```python
from build123d import *

# Parameters (mm, degrees)
BOSS_EXTRUDE1_DEPTH = 261.8
CUT_EXTRUDE1_DEPTH  = 4001.062499512


with BuildPart() as part:
    # Sketch1 → Boss-Extrude1 (new body)
    with BuildSketch(Plane.XY.offset(4000)):
        with BuildLine():
            Line((10, 3.138), (10, 8.5))
            ThreePointArc((10, 8.5), (9.560660172, 9.560660172), (8.5, 10))
            Line((8.5, 10), (3.138, 10))
            ThreePointArc((3.138, 10), (2.778789755, 9.851210245), (2.63, 9.492))
            Line((2.63, 9.492), (2.63, 9.008))
            ThreePointArc((2.63, 9.008), (2.778789755, 8.648789755), (3.138, 8.5))
            Line((3.138, 8.5), (5.487, 8.5))
            ThreePointArc((5.487, 8.5), (5.846210245, 8.351210245), (5.995, 7.992))
            Line((5.995, 7.992), (5.995, 7.266080661))
            ThreePointArc((5.995, 7.266080661), (5.956330803, 7.071677478), (5.846210245, 6.906870417))
            Line((5.846210245, 6.906870417), (2.743129583, 3.803789755))
            ThreePointArc((2.743129583, 3.803789755), (2.578322522, 3.693669197), (2.383919339, 3.655))
            Line((2.383919339, 3.655), (-2.383919339, 3.655))
            ThreePointArc((-2.383919339, 3.655), (-2.578322522, 3.693669197), (-2.743129583, 3.803789755))
            Line((-2.743129583, 3.803789755), (-5.846210245, 6.906870417))
            ThreePointArc((-5.846210245, 6.906870417), (-5.956330803, 7.071677478), (-5.995, 7.266080661))
            Line((-5.995, 7.266080661), (-5.995, 7.992))
            ThreePointArc((-5.995, 7.992), (-5.846210245, 8.351210245), (-5.487, 8.5))
            Line((-5.487, 8.5), (-3.138, 8.5))
            ThreePointArc((-3.138, 8.5), (-2.778789755, 8.648789755), (-2.63, 9.008))
            Line((-2.63, 9.008), (-2.63, 9.492))
            ThreePointArc((-2.63, 9.492), (-2.778789755, 9.851210245), (-3.138, 10))
            Line((-3.138, 10), (-8.5, 10))
            ThreePointArc((-8.5, 10), (-9.560660172, 9.560660172), (-10, 8.5))
            Line((-10, 8.5), (-10, 3.138))
            ThreePointArc((-10, 3.138), (-9.851210245, 2.778789755), (-9.492, 2.63))
            Line((-9.492, 2.63), (-9.008, 2.63))
            ThreePointArc((-9.008, 2.63), (-8.648789755, 2.778789755), (-8.5, 3.138))
            Line((-8.5, 3.138), (-8.5, 5.487))
            ThreePointArc((-8.5, 5.487), (-8.351210245, 5.846210245), (-7.992, 5.995))
            Line((-7.992, 5.995), (-7.266080661, 5.995))
            ThreePointArc((-7.266080661, 5.995), (-7.071677478, 5.956330803), (-6.906870417, 5.846210245))
            Line((-6.906870417, 5.846210245), (-3.803789755, 2.743129583))
            ThreePointArc((-3.803789755, 2.743129583), (-3.693669197, 2.578322522), (-3.655, 2.383919339))
            Line((-3.655, 2.383919339), (-3.655, -2.383919339))
            ThreePointArc((-3.655, -2.383919339), (-3.693669197, -2.578322522), (-3.803789755, -2.743129583))
            Line((-3.803789755, -2.743129583), (-6.906870417, -5.846210245))
            ThreePointArc((-6.906870417, -5.846210245), (-7.071677478, -5.956330803), (-7.266080661, -5.995))
            Line((-7.266080661, -5.995), (-7.992, -5.995))
            ThreePointArc((-7.992, -5.995), (-8.351210245, -5.846210245), (-8.5, -5.487))
            Line((-8.5, -5.487), (-8.5, -3.138))
            ThreePointArc((-8.5, -3.138), (-8.648789755, -2.778789755), (-9.008, -2.63))
            Line((-9.008, -2.63), (-9.492, -2.63))
            ThreePointArc((-9.492, -2.63), (-9.851210245, -2.778789755), (-10, -3.138))
            Line((-10, -3.138), (-10, -8.5))
            ThreePointArc((-10, -8.5), (-9.560660172, -9.560660172), (-8.5, -10))
            Line((-8.5, -10), (-3.138, -10))
            ThreePointArc((-3.138, -10), (-2.778789755, -9.851210245), (-2.63, -9.492))
            Line((-2.63, -9.492), (-2.63, -9.008))
            ThreePointArc((-2.63, -9.008), (-2.778789755, -8.648789755), (-3.138, -8.5))
            Line((-3.138, -8.5), (-5.487, -8.5))
            ThreePointArc((-5.487, -8.5), (-5.846210245, -8.351210245), (-5.995, -7.992))
            Line((-5.995, -7.992), (-5.995, -7.266080661))
            ThreePointArc((-5.995, -7.266080661), (-5.956330803, -7.071677478), (-5.846210245, -6.906870417))
            Line((-5.846210245, -6.906870417), (-2.743129583, -3.803789755))
            ThreePointArc((-2.743129583, -3.803789755), (-2.578322522, -3.693669197), (-2.383919339, -3.655))
            Line((-2.383919339, -3.655), (2.383919339, -3.655))
            ThreePointArc((2.383919339, -3.655), (2.578322522, -3.693669197), (2.743129583, -3.803789755))
            Line((2.743129583, -3.803789755), (5.846210245, -6.906870417))
            ThreePointArc((5.846210245, -6.906870417), (5.956330803, -7.071677478), (5.995, -7.266080661))
            Line((5.995, -7.266080661), (5.995, -7.992))
            ThreePointArc((5.995, -7.992), (5.846210245, -8.351210245), (5.487, -8.5))
            Line((5.487, -8.5), (3.138, -8.5))
            ThreePointArc((3.138, -8.5), (2.778789755, -8.648789755), (2.63, -9.008))
            Line((2.63, -9.008), (2.63, -9.492))
            ThreePointArc((2.63, -9.492), (2.778789755, -9.851210245), (3.138, -10))
            Line((3.138, -10), (8.5, -10))
            ThreePointArc((8.5, -10), (9.560660172, -9.560660172), (10, -8.5))
            Line((10, -8.5), (10, -3.138))
            ThreePointArc((10, -3.138), (9.851210245, -2.778789755), (9.492, -2.63))
            Line((9.492, -2.63), (9.008, -2.63))
            ThreePointArc((9.008, -2.63), (8.648789755, -2.778789755), (8.5, -3.138))
            Line((8.5, -3.138), (8.5, -5.487))
            ThreePointArc((8.5, -5.487), (8.351210245, -5.846210245), (7.992, -5.995))
            Line((7.992, -5.995), (7.266080661, -5.995))
            ThreePointArc((7.266080661, -5.995), (7.071677478, -5.956330803), (6.906870417, -5.846210245))
            Line((6.906870417, -5.846210245), (3.803789755, -2.743129583))
            ThreePointArc((3.803789755, -2.743129583), (3.693669197, -2.578322522), (3.655, -2.383919339))
            Line((3.655, -2.383919339), (3.655, 2.383919339))
            ThreePointArc((3.655, 2.383919339), (3.693669197, 2.578322522), (3.803789755, 2.743129583))
            Line((3.803789755, 2.743129583), (6.906870417, 5.846210245))
            ThreePointArc((6.906870417, 5.846210245), (7.071677478, 5.956330803), (7.266080661, 5.995))
            Line((7.266080661, 5.995), (7.992, 5.995))
            ThreePointArc((7.992, 5.995), (8.351210245, 5.846210245), (8.5, 5.487))
            Line((8.5, 5.487), (8.5, 3.138))
            ThreePointArc((8.5, 3.138), (8.648789755, 2.778789755), (9.008, 2.63))
            Line((9.008, 2.63), (9.492, 2.63))
            ThreePointArc((9.492, 2.63), (9.851210245, 2.778789755), (10, 3.138))
        make_face()
        with BuildLine():
            Line((-2.124900844, -2.304505966), (-2.304505966, -2.124900844))
            ThreePointArc((-2.304505966, -2.124900844), (-2.505938017, -1.356467811), (-1.935133506, -0.803976718))
            ThreePointArc((-1.935133506, -0.803976718), (-2.0955, 0), (-1.935133506, 0.803976718))
            ThreePointArc((-1.935133506, 0.803976718), (-2.505938017, 1.356467811), (-2.304505966, 2.124900844))
            Line((-2.304505966, 2.124900844), (-2.124900844, 2.304505966))
            ThreePointArc((-2.124900844, 2.304505966), (-1.356467811, 2.505938017), (-0.803976718, 1.935133506))
            ThreePointArc((-0.803976718, 1.935133506), (0, 2.0955), (0.803976718, 1.935133506))
            ThreePointArc((0.803976718, 1.935133506), (1.356467811, 2.505938017), (2.124900844, 2.304505966))
            Line((2.124900844, 2.304505966), (2.304505966, 2.124900844))
            ThreePointArc((2.304505966, 2.124900844), (2.505938017, 1.356467811), (1.935133506, 0.803976718))
            ThreePointArc((1.935133506, 0.803976718), (2.0955, 0), (1.935133506, -0.803976718))
            ThreePointArc((1.935133506, -0.803976718), (2.505938017, -1.356467811), (2.304505966, -2.124900844))
            Line((2.304505966, -2.124900844), (2.124900844, -2.304505966))
            ThreePointArc((2.124900844, -2.304505966), (1.356467811, -2.505938017), (0.803976718, -1.935133506))
            ThreePointArc((0.803976718, -1.935133506), (0, -2.0955), (-0.803976718, -1.935133506))
            ThreePointArc((-0.803976718, -1.935133506), (-1.356467811, -2.505938017), (-2.124900844, -2.304505966))
        make_face(mode=Mode.SUBTRACT)
    extrude(amount=-BOSS_EXTRUDE1_DEPTH)

    # Sketch2 → Cut-Extrude1 (cut, through all)
    with BuildSketch(Plane.XZ.offset(10)):
        Polygon((10, 4000), (-10, 3995.213189756), (-10, 4000), align=None)
        Polygon((10, 3738.2), (10, 3742.986810244), (-10, 3738.2), align=None)
    extrude(amount=-CUT_EXTRUDE1_DEPTH, mode=Mode.SUBTRACT)


solid = part.part
```
Source: CAD feature listing. Evaluate the final solid. Frame: model axes, mm. A direction names the side the tool comes from. Round coordinates to 2 decimals unless told otherwise and drop trailing zeros. Use a Markdown table: item, result. Add a question column.
1. Ray query, line 1 along X through (y, z) = (-4.75, 3887); line 2 along Y through (x, z) = (1, 3956) (3 decimals); line 3 along X through (y, z) = (-8, 3987). Return the intervals inside material, ascending. Write a range as [from, to].
2. Contact query for flat-ended pins moving along their axis: pin 1 (5 mm diameter, centred on x = -3, y = 6.5, fed in from -Z); pin 2 (0.5 mm diameter, centred on y = -9.5, z = 3834.5, fed in from +X); pin 3 (1 mm diameter, centred on x = 2, z = 3772, fed in from +Y). Output: stop coordinate, or through.
3. Pull-direction query (X, two-part tool) for faces 1 (the flat face through (0, 3.655, 3871)), 2 (the flat face through (3.655, 0, 3872)), 3 (the flat face through (-6, 10, 3870)); classes: +X half, -X half, draft (parallel to the pull), parting line (faces both ways), or undercut.
4. Set-up query: faces 4 (the flat face through (10, 6, 3873)), 5 (the flat face through (-3.655, 0, 3870)), 6 (the flat face through (0, -3.655, 3871)). Return all of +Z, -Z, +X, -X, +Y, -Y with unobstructed straight access to the full face (end or side cutting, diameter ignored); none if empty.
Solution:
| question | item | result |
|---|---|---|
| 1 | line 1 | x = [-10, -8.5], [-5.81, -3.69], [3.69, 5.81], [8.5, 10] |
| 1 | line 2 | y = [-3.655, -2.292], [2.292, 3.655] |
| 1 | line 3 | x = [-10, -5.99], [5.99, 10] |
| 2 | pin 1 | stops at z = 3739.28 |
| 2 | pin 2 | stops at x = 9.8 |
| 2 | pin 3 | stops at y = 3.67 |
| 3 | face 1 | undercut |
| 3 | face 2 | +X half |
| 3 | face 3 | draft |
| 4 | face 4 | +Z, -Z, +X, +Y, -Y |
| 4 | face 5 | +Z, -Z, -X |
| 4 | face 6 | +Z, -Z, -Y |
